Build history of the part. All positions in model axes, mm. A direction names the side the tool comes from. Round coordinates to 2 decimals unless told otherwise and drop trailing zeros. Order: outer loops, then holes, each group sorted by start corner. A loop starts at its lowest first (then second) coordinate and runs counter-clockwise, first axis right, second up. Notation, with made-up numbers: (8.25, -15.75) -> (21.25, -15.75) arc R35 cw to (21.25, 20.25) -> close; hole circle Ø8 at (75, 30). An arc over 180 degrees is marked (long way). Use a Markdown table: item, result. Add a question column.
Item 1: Slice it at C-C, the plane z = -30.5. Give the cut face in (x, y).
Item 2: Two-plate mould, pull along Y, no slides. Class faces 1 (the face through (-22, -25.4, 32)), 2 (the face through (-21.76, -11.41, 37.39)), 3 (the face through (34, 73.861, 36)): released by +Y, released by -Y, zero draft, split by the parting line, or undercut.
Item 3: Slice it at A-A, the plane y = -40.5. Give the cut face in (x, z).
Item 4: Pin check, flat tips, straight feed: pin 1 (3 mm diameter, centred on y = -10.5, z = 35, fed in from -X); pin 2 (12 mm diameter, centred on x = -32, y = -22.5, fed in from -Z); pin 3 (12.5 mm diameter, centred on x = -3, z = 37.5, fed in from -Y). Stop position of each tip, or through.
Item 5: 3-axis set-ups, long thin cutter, end or side, ignore diameter. For faces 4 (the face through (-20.47, -21.58, 10.31)), 5 (the face through (-22, 0, 32)), 6 (the face through (-20.473, -21.581, 53.205)), 7 (the face through (-20.473, -3.819, 53.205)): which of +Z, -Z, +X, -X, +Y, -Y reach the whole face in a straight line?
Item 6: Probe L1, parallel to X at y = 63.5, z = -54; L2, parallel to Z at x = 3.5, y = -20.5. List the from-to ranges inside material, lowest first.
Item 7: Slice it at D-D, the plane y = -5. Give the cut face in (x, z).
from build123d import *

# Parameters (mm, degrees)
F0_W     = 91.694
F0_H     = 50.1397587359
F1_DEPTH = 25.4
F2_R     = 12.69999
F4_D     = 6.35
F5_W     = 135.6123574078
F5_H     = 257.5739622116
F6_DEPTH = 19.05


# Not quite as in the source:
# - a fillet or chamfer is up to 0.001 mm smaller than in the source, because OpenCascade refuses the exact size


with BuildPart() as f1:
    # F0 (on Front) → F1 (new body)
    with BuildSketch(Plane.XZ):
        with Locations((-21.1153341503, 31.7568909377)):
            Rectangle(F0_W, F0_H)
    extrude(amount=F1_DEPTH)

    # F2 (radius 12.7 in the source; OpenCascade refuses exactly that, so slightly less here)
    f2_edges = [f1.edges().sort_by_distance(p)[0] for p in [
        (-21.115334, -25.4, 56.82677),
        (-21.115334, -25.4, 6.687012),
        (-21.115334, 0, 56.82677),
        (-21.115334, 0, 6.687012),
    ]]
    fillet(f2_edges, radius=F2_R)

    # F4 (through all)
    with Locations(Plane.YZ.offset(24.7316658497)):
        with Locations((-11.8228401989, 34.2414677143)):
            Hole(F4_D / 2)

    # F5 (on face) → F6 (join)
    with BuildSketch(Plane.YZ.offset(24.7316658497)):
        with Locations((6.0548242182, 38.2600277662)):
            Rectangle(F5_W, F5_H)
    extrude(amount=F6_DEPTH)


solid = f1.part
Check sheet entries:
| question | item | result |
|---|---|---|
| 1 | outline | (24.73, -61.75) -> (43.78, -61.75) -> (43.78, 73.86) -> (24.73, 73.86) -> close |
| 2 | face 1 | released by -Y |
| 2 | face 2 | undercut |
| 2 | face 3 | released by +Y |
| 3 | outline | (24.73, -90.53) -> (43.78, -90.53) -> (43.78, 167.05) -> (24.73, 167.05) -> close |
| 4 | pin 1 | x = 24.73 |
| 4 | pin 2 | z = 7.27 |
| 4 | pin 3 | y = -25.4 |
| 5 | face 4 | -Z, -X, -Y |
| 5 | face 5 | +Z, -Z, -X, +Y |
| 5 | face 6 | +Z, -X, -Y |
| 5 | face 7 | +Z, -X, +Y |
| 6 | L1 | 24.73 to 43.78 |
| 6 | L2 | 9.36 to 54.15 |
| 7 | outline | (-66.96, 9.29) -> (24.73, 9.29) -> (24.73, -90.53) -> (43.78, -90.53) -> (43.78, 167.05) -> (24.73, 167.05) -> (24.73, 54.23) -> (-66.96, 54.23) -> close |
